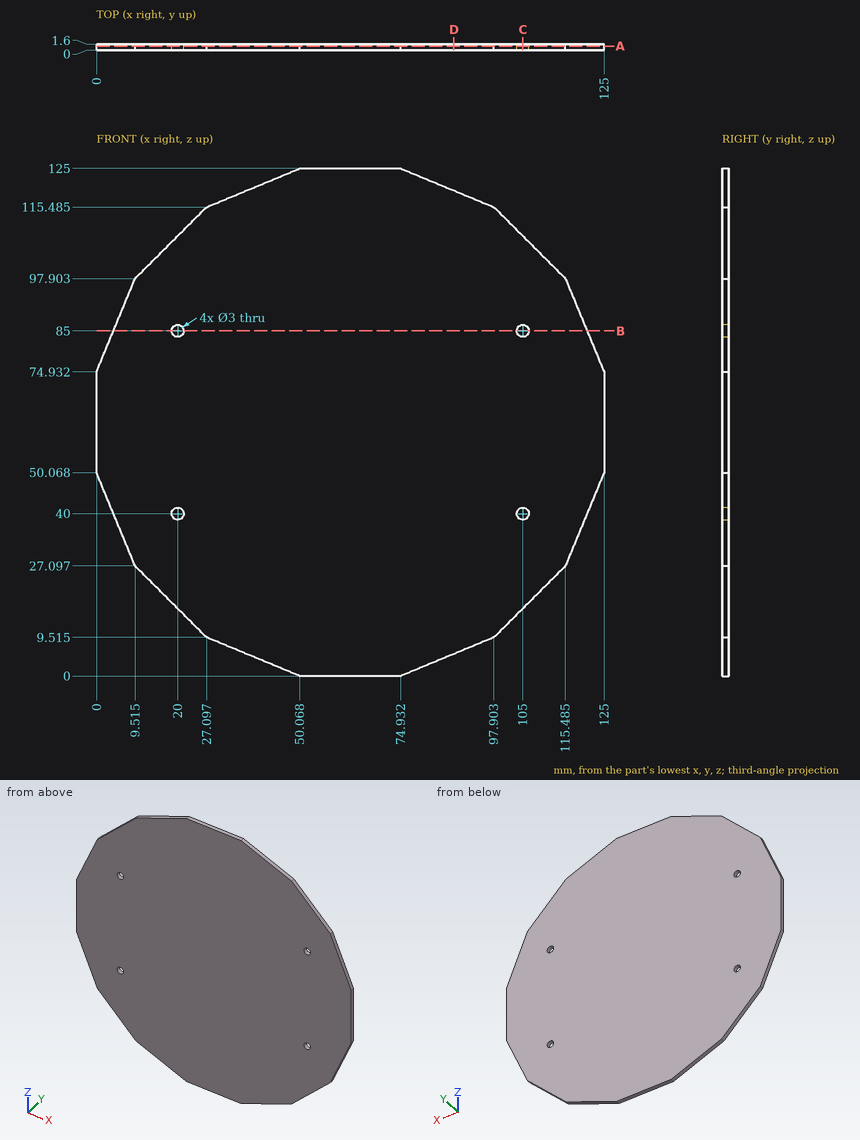
Part print with two shaded views. Sizes in mm from the minimum x, y, z corner. Coordinates: 2 decimals unless noted, no trailing zeros. Order: outer loops, then holes, each group sorted by start corner. A loop starts at its lowest first (then second) coordinate and runs counter-clockwise, first axis right, second up. Notation, with made-up numbers: M -39.5,-19 L -26.5,-19 A26 ccw -26.5,4 Z; hole C 88.5,18 d7. An arc over 180 degrees is marked long. Use a Markdown table: item, result.
(1) Flat gauge pins, fed straight in: pin 1 (3.5 mm diameter, centred on x = 105, z = 40, fed in from -Y); pin 2 (2.5 mm diameter, centred on x = 105, z = 85, fed in from -Y). Where does each tip first touch, or does it go through?
A:
| item | result |
|---|---|
| pin 1 | stops at y = 0 |
| pin 2 | passes through |
(2) Cut at A-A on y = 1.05. Write the cut outline in (x, z) (1 decimal), then the cut area to 3 significant figures.
A:
| item | result |
|---|---|
| outline | M 0,50.1 L 9.5,27.1 L 27.1,9.5 L 50.1,0 L 74.9,0 L 97.9,9.5 L 115.5,27.1 L 125,50.1 L 125,74.9 L 115.5,97.9 L 97.9,115.5 L 74.9,125 L 50.1,125 L 27.1,115.5 L 9.5,97.9 L 0,74.9 Z; hole C 20,40 d3; hole C 20,85 d3; hole C 105,40 d3; hole C 105,85 d3 |
| area | 12,400 mm^2 |
(3) Cut at D-D on x = 88. Write the cut outline in (y, z).
A:
| item | result |
|---|---|
| outline | M 0,5.41 L 1.6,5.41 L 1.6,119.59 L 0,119.59 Z |
(4) Cut at C-C on x = 105. Write the cut outline in (y, z), then the cut area to 3 significant figures.
A:
| item | result |
|---|---|
| outline | M 0,16.61 L 1.6,16.61 L 1.6,38.5 L 0,38.5 Z; M 0,41.5 L 1.6,41.5 L 1.6,83.5 L 0,83.5 Z; M 0,86.5 L 1.6,86.5 L 1.6,108.39 L 0,108.39 Z |
| area | 137 mm^2 |
(5) Probe L1, parallel to X at y = 0.35, z = 85; L2, parallel to Z at x = 105, y = 0.4; L3, parallel to Z at x = 9.5, y = 0.9 (1 decimal). List the from-to ranges inside material, lowest first.
A:
| item | result |
|---|---|
| L1 | x = 4.17 to 18.5, 21.5 to 103.5, 106.5 to 120.83 |
| L2 | z = 16.61 to 38.5, 41.5 to 83.5, 86.5 to 108.39 |
| L3 | z = 27.1 to 97.9 |
(6) Cut at B-B on z = 85. Write the cut outline in (x, y), then the cut area to 3 significant figures.
A:
| item | result |
|---|---|
| outline | M 4.17,0 L 18.5,0 L 18.5,1.6 L 4.17,1.6 Z; M 21.5,0 L 103.5,0 L 103.5,1.6 L 21.5,1.6 Z; M 106.5,0 L 120.83,0 L 120.83,1.6 L 106.5,1.6 Z |
| area | 177 mm^2 |
